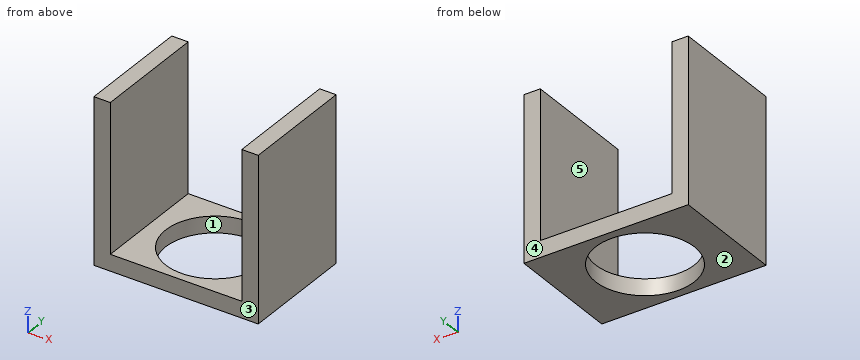
```python
from build123d import *

# Parameters (mm, degrees)
ESQUISSE1_W             = 80
ESQUISSE1_H             = 70
BOSS_EXTRU_2_DEPTH      = 10
ESQUISSE1_4_W           = 10
ESQUISSE1_4_H           = 70
BOSS_EXTRU_3_DEPTH      = 100
ESQUISSE4_R             = 30
ENL_V_MAT_EXTRU_1_DEPTH = 10


with BuildPart() as part:
    # Esquisse1 → Boss.-Extru.2 (new body)
    with BuildSketch(Plane.XY):
        with Locations((-50, 35)):
            Rectangle(ESQUISSE1_W, ESQUISSE1_H)
    extrude(amount=BOSS_EXTRU_2_DEPTH)

    # Esquisse1<4> → Boss.-Extru.3 (add)
    with BuildSketch(Plane.XY):
        with Locations((-5, 35)):
            Rectangle(ESQUISSE1_4_W, ESQUISSE1_4_H)
        with Locations((-95, 35)):
            Rectangle(ESQUISSE1_4_W, ESQUISSE1_4_H)
    extrude(amount=BOSS_EXTRU_3_DEPTH)

    # Esquisse4 → Enlèv. mat.-Extru.1 (cut)
    with BuildSketch(Plane.XY):
        with Locations((-50, 35)):
            Circle(ESQUISSE4_R)
    extrude(amount=ENL_V_MAT_EXTRU_1_DEPTH, mode=Mode.SUBTRACT)


solid = part.part
```
Input: part model. Units: mm. Frame: model coordinates. Face numbers are marked on the shaded views. A direction names the side the tool comes from. Give positions to 0.01 mm unless a question says otherwise; leave off trailing zeros. Loops run counter-clockwise (first coordinate to the right, second up) from the corner with the lowest first, then second, coordinate; pieces in that order, holes last.
1) Section query D-D on y = 25. Return the cut outline in (x, z).
A:
outline: (-100, 0) - (-78.28, 0) - (-78.28, 10) - (-90, 10) - (-90, 100) - (-100, 100) - close; (-21.72, 0) - (0, 0) - (0, 100) - (-10, 100) - (-10, 10) - (-21.72, 10) - close
2) Section query B-B on y = 35. Return the cut outline in (x, z).
A:
outline: (-100, 0) - (-80, 0) - (-80, 10) - (-90, 10) - (-90, 100) - (-100, 100) - close; (-20, 0) - (0, 0) - (0, 100) - (-10, 100) - (-10, 10) - (-20, 10) - close
3) Section query C-C on z = 52. Return the cut outline in (x, y), and give its area (3 significant figures).
A:
outline: (-100, 0) - (-90, 0) - (-90, 70) - (-100, 70) - close; (-10, 0) - (0, 0) - (0, 70) - (-10, 70) - close
area: 1,400 mm2
4) Section query A-A on x = -50. Return the cut outline in (y, z).
A:
outline: (0, 0) - (5, 0) - (5, 10) - (0, 10) - close; (65, 0) - (70, 0) - (70, 10) - (65, 10) - close
5) Line query: L1, parallel to Y at x = -50, z = 4.75; L2, parallel to X at y = 24.5, z = 41.5; L3, parallel to Y at x = -66, z = 5. Output: solid intervals per line, ascending.
A:
L1: y = 0 to 5, 65 to 70
L2: x = -100 to -90, -10 to 0
L3: y = 0 to 9.62, 60.38 to 70
6) Mould query, pull axis Y, two halves, no side actions, for the marked faces 1, 2 and 3. Classes: released by +Y, released by -Y, zero draft, split by the parting line, or undercut.
A:
face 1: undercut
face 2: zero draft
face 3: released by -Y
7) Reachability of the marked faces 4 and 5 from +Z, -Z, +X, -X, +Y, -Y: full face, straight path, thin tool, end or side. Return the list, or none.
A:
face 4: +Z, -Z, +X, -X, +Y
face 5: +Z, +Y, -Y
